Source: CAD feature listing. Evaluate the final solid. Frame: model axes, mm. A direction names the side the tool comes from. Give positions to 0.01 mm unless a question says otherwise; leave off trailing zeros. Write each loop counter-clockwise with the first axis right and the second up, starting at its lowest first coordinate (ties: lowest second). Pieces come first, ordered by that corner, then holes. Notation, with made-up numbers: (77.5, 70.5) -> (81.5, 70.5) arc R20 cw to (81.5, 83.5) -> close; hole circle Ø3 at (-33, -19.5). An arc over 180 degrees is marked (long way). Answer as a JSON object with one key per item and string values. Group by question number.
Item 1: Pull-direction query (X, two-part tool) for faces 5 (the face through (12, 1, -33)), 6 (the face through (-15.5, 1, -31)), 7 (the face through (-9.5, 1, -32)), 8 (the face through (0, 1, -30)); classes: pulls with the +X half, pulls with the -X half, needs draft (parallel to the pull), parting line crosses it, or undercut.
Item 2: First-contact query: pin 1 Ø1.5 at (x, y) = (22, 2) entering from +Z; pin 2 Ø0.9 at (y, z) = (1.5, -31) entering from -X; pin 3 Ø0.9 at (y, z) = (2, 2) entering from +X. Flat tips, straight axial feed; report the tip coordinate or a pass-through.
Item 3: Access query for faces 1 (the face through (-20, 1, -30)), 2 (the face through (9.5, 1, -31)), 3 (the face through (15.5, 1, 1)), 4 (the face through (20, 1, -30)). Directions: +Z, -Z, +X, -X, +Y, -Y. A direction counts if a zero-diameter tool reaches every point of the face in a straight line with its end or side. Return the directions, or none.
Item 4: Section query A-A on y = 0.8. Return the cut outline in (x, z).
Item 5: Ray query, probe 1 along X at (y, z) = (2.25, 0.5); probe 2 along Z at (x, y) = (7, 0.5). Return the intervals inside material, ascending. Write a range as from..to.
Item 6: Section query B-B on x = -18. Return the cut outline in (y, z), plus the area to 3 significant figures.
Autodesk Inventor part; units mm, degrees
ref_plane "YZ Plane" through (0, 0, 0) normal (1, 0, 0) x (0, 1, 0)
ref_plane "XZ Plane" through (0, 0, 0) normal (0, 1, 0) x (-1, 0, 0)
ref_plane "XY Plane" through (0, 0, 0) normal (0, 0, 1) x (1, 0, 0)
sketch "Sketch1" plane through (0, 0, 0) normal (0, 1, 0) x (-1, 0, 0)
  line L0 (-15.5, 0) -> (-15.5, 3)
  line L1 (-15.5, 3) -> (-9.5, 3)
  line L2 (-9.5, 3) -> (-9.5, 0)
  line L3 (15.5, 0) -> (15.5, 3)
  line L4 (15.5, 3) -> (9.5, 3)
  line L5 (9.5, 3) -> (9.5, 0)
  line L6 (-15.5, 0) -> (-15.5, 3)
  line L7 (-15.5, 3) -> (-9.5, 3)
  line L8 (-9.5, 3) -> (-9.5, 0)
  line L9 (15.5, 0) -> (15.5, 3)
  line L10 (15.5, 3) -> (9.5, 3)
  line L11 (9.5, 3) -> (9.5, 0)
  line L12 (-25, 0) -> (-15.5, 0)
  line L13 (-9.5, 0) -> (9.5, 0)
  line L14 (15.5, 0) -> (25, 0)
  line L15 (25, 0) -> (25, -30)
  line L16 (-25, 0) -> (-25, -30)
  line L17 (25, -30) -> (15.5, -30)
  line L18 (15.5, -30) -> (15.5, -33)
  line L19 (15.5, -33) -> (9.5, -33)
  line L20 (9.5, -33) -> (9.5, -30)
  line L21 (9.5, -30) -> (-9.5, -30)
  line L22 (-9.5, -30) -> (-9.5, -33)
  line L23 (-9.5, -33) -> (-15.5, -33)
  line L24 (-15.5, -33) -> (-15.5, -30)
  line L25 (-15.5, -30) -> (-25, -30)
  point P0 (0, 0)
  dimension "d3" = 3
  dimension "d4" = 6
  dimension "d7" = 3
  dimension "d8" = 6
  dimension "d12" = 3
  dimension "d13" = 6
  dimension "d16" = 3
  dimension "d17" = 6
  dimension "d19" = 30
  dimension "d20" = 30
  dimension "d21" = 3
extrude "Extrusion1" add sketch "Sketch1" along normal blind 3
properties part number "Ball Capture Zone Cover plate" material "Rubber"
Worked answers:
{
 "1": {"face 5": "needs draft", "face 6": "pulls with the -X half", "face 7": "undercut", "face 8": "undercut"},
 "2": {"pin 1": "z = 0", "pin 2": "x = -15.5", "pin 3": "x = 15.5"},
 "3": {"face 1": "-Z, -X, +Y, -Y", "face 2": "-Z, +Y, -Y", "face 3": "+Z, +X, +Y, -Y", "face 4": "-Z, +X, +Y, -Y"},
 "4": {"outline": "(-25, -30) -> (-15.5, -30) -> (-15.5, -33) -> (-9.5, -33) -> (-9.5, -30) -> (9.5, -30) -> (9.5, -33) -> (15.5, -33) -> (15.5, -30) -> (25, -30) -> (25, 0) -> (15.5, 0) -> (15.5, 3) -> (9.5, 3) -> (9.5, 0) -> (-9.5, 0) -> (-9.5, 3) -> (-15.5, 3) -> (-15.5, 0) -> (-25, 0) -> close"},
 "5": {"probe 1": "-15.5..-9.5, 9.5..15.5", "probe 2": "-30..0"},
 "6": {"outline": "(0, -30) -> (3, -30) -> (3, 0) -> (0, 0) -> close", "area": "90.0 mm^2"}
}
